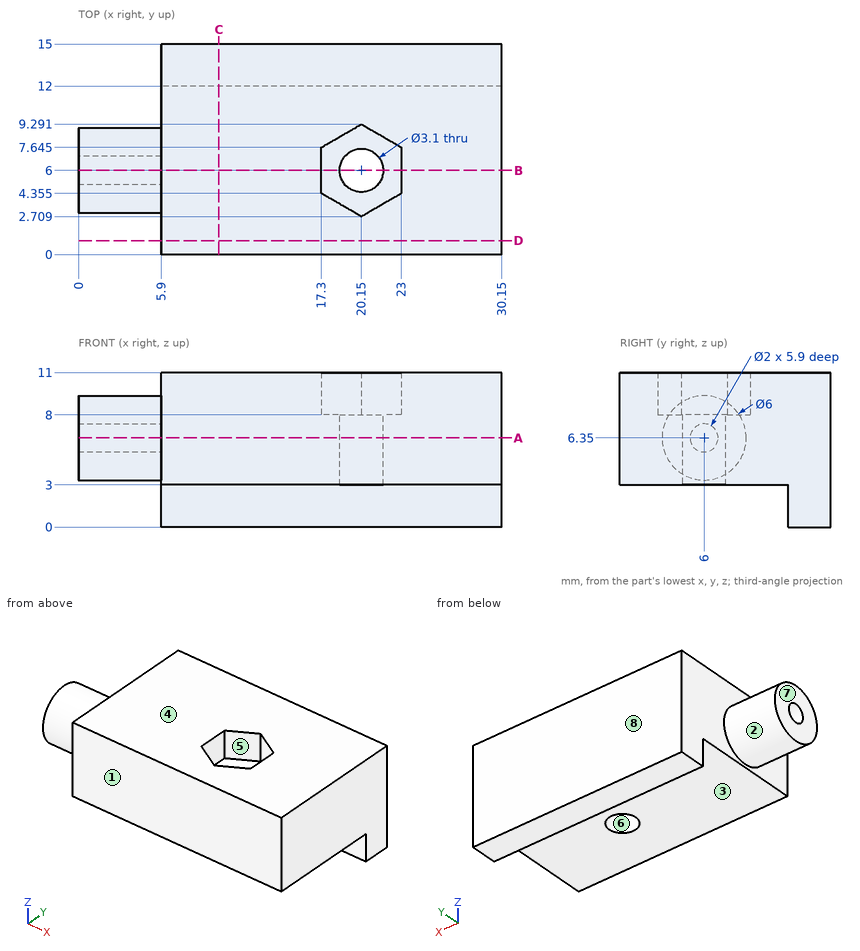
Geometry: see drawing. Coordinates: mm, zero at the bounding-box minimum. A direction names the side the tool comes from. Round coordinates to 2 decimals unless told otherwise and drop trailing zeros. Write each loop counter-clockwise with the first axis right and the second up, starting at its lowest first coordinate (ties: lowest second). Pieces come first, ordered by that corner, then holes.
Item 1: Section query C-C (x = 10). Return loops of the section in (y, z), plus the area to 3 significant figures.
Item 2: Section query B-B (y = 6). Return loops of the section in (x, z).
Item 3: Section query A-A (z = 6.35). Return loops of the section in (x, y).
Item 4: Material intervals for L1, parallel to Z at x = 1.85, y = 6; L2, parallel to X at y = 6, z = 5.85; L3, parallel to Y at x = 20.15, z = 4.1, sorted ascending.
Item 5: Set-up query: the marked faces 1, 2, 3, 4 and 5. Return all of +Z, -Z, +X, -X, +Y, -Y with unobstructed straight access to the full face (end or side cutting, diameter ignored); none if empty.
Item 6: Pin query (flat end, axial travel): P1, Ø1, axis at y = 8.5, z = 2, coming from the -X side; P2, Ø1.5, axis at x = 14.5, z = 1.5, coming from the -Y side; P3, Ø3.5, axis at x = 20.15, y = 6, coming from the +Z side. Return the tip coordinate at first contact, or that it passes through.
Item 7: Mould query, pull axis Y, two halves, no side actions, for the marked faces 6, 7 and 8. Classes: +Y half, -Y half, draft (parallel to the pull), parting line (faces both ways), or undercut.
Item 8: Section query D-D (y = 1). Return loops of the section in (x, z), plus the area to 3 significant figures.
Completed:
1. outline: (0, 3) - (12, 3) - (12, 0) - (15, 0) - (15, 11) - (0, 11) - close
1. area: 129 mm2
2. outline: (0, 3.35) - (5.9, 3.35) - (5.9, 3) - (18.6, 3) - (18.6, 8) - (17.3, 8) - (17.3, 11) - (5.9, 11) - (5.9, 9.35) - (0, 9.35) - (0, 7.35) - (5.9, 7.35) - (5.9, 5.35) - (0, 5.35) - close; (21.7, 3) - (30.15, 3) - (30.15, 11) - (23, 11) - (23, 8) - (21.7, 8) - close
3. outline: (0, 3) - (5.9, 3) - (5.9, 0) - (30.15, 0) - (30.15, 15) - (5.9, 15) - (5.9, 9) - (0, 9) - (0, 7) - (5.9, 7) - (5.9, 5) - (0, 5) - close; hole circle Ø3.1 at (20.15, 6)
4. L1: z = 3.35 to 5.35, 7.35 to 9.35
4. L2: x = 5.9 to 18.6, 21.7 to 30.15
4. L3: y = 0 to 4.45, 7.55 to 15
5. face 1: +Z, -Z, +X, -X, -Y
5. face 2: -X
5. face 3: -Z, +X, -X, -Y
5. face 4: +Z, +X, -X, +Y, -Y
5. face 5: +Z
6. P1: passes through
6. P2: stops at y = 12
6. P3: stops at z = 8
7. face 6: undercut
7. face 7: draft
7. face 8: +Y half
8. outline: (5.9, 3) - (30.15, 3) - (30.15, 11) - (5.9, 11) - close
8. area: 194 mm2
